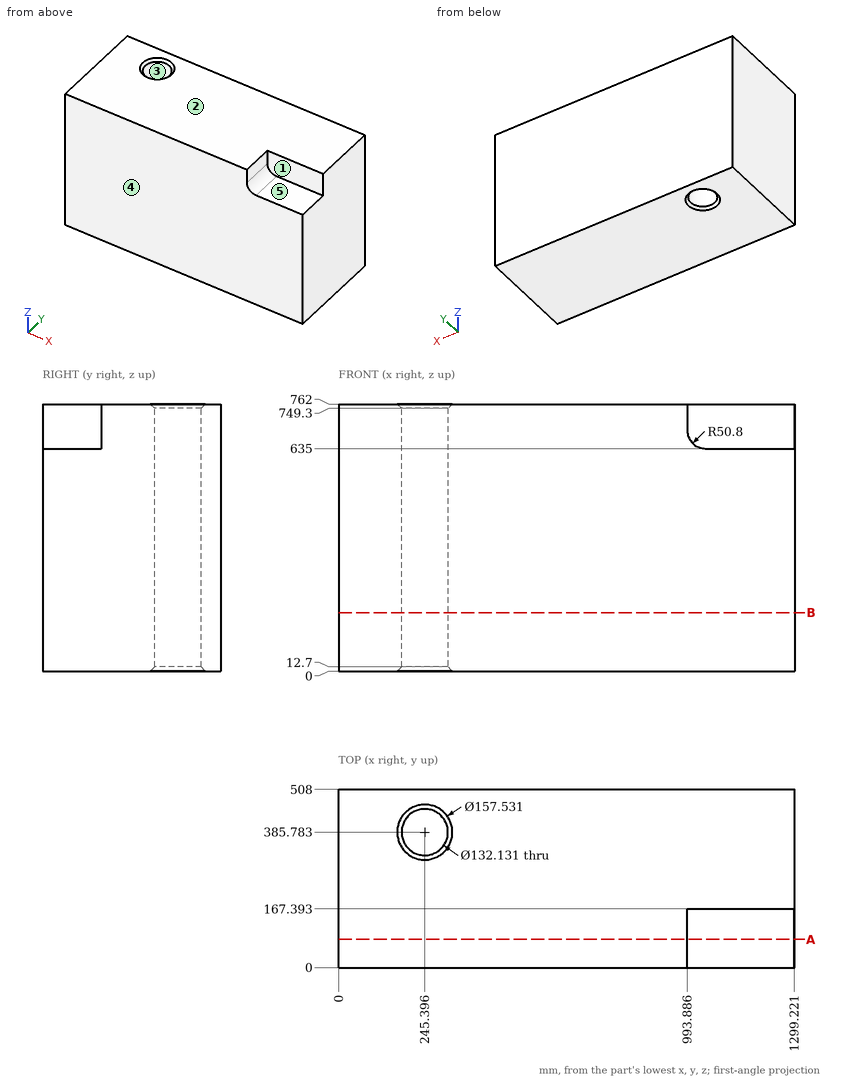
Design review of the part shown in the three views and the two pictorial views. Dimensions are in mm from the part's minimum x, y and z. A direction names the side the tool comes from. Coordinates: 2 decimals unless noted, no trailing zeros. Write each loop counter-clockwise with the first axis right and the second up, starting at its lowest first coordinate (ties: lowest second). Pieces come first, ordered by that corner, then holes.
(1) The part is to be moulded in two halves that separate along Y. For the marked faces 3, 4 and 5, say which applies: +Y half, -Y half, draft (parallel to the pull), parting line (faces both ways), or undercut.
(2) Wall thickness on probe 1 along Z at (x, y) = (1150.5, 45); probe 2 along X at (y, z) = (400, 229); probe 3 along X at (y, z) = (42, 704): over which ranges is each line inside the solid? List them lowest first.
(3) For pin 1 Ø5 at (y, z) = (113, 684.5) entering from -X; pin 2 Ø23 at (y, z) = (56, 739.5) entering from +X, all flat-tipped, find the tip position at first contact; note any pin that passes through.
(4) Add section B-B on z = 167. Give the boundary of the cut face in (x, y) (1 decimal), then the cut area to 3 significant figures.
(5) Add section A-A on y = 80.5. Give the boundary of the cut face in (x, z), then the cut area to 3 significant figures.
(6) Tool access review of the marked faces 1 and 2: name each direction out of +Z, -Z, +X, -X, +Y, -Y from which nothing blocks a thin tool from reaching the whole face with its end or side.
Answer sheet:
1. face 3: undercut
1. face 4: -Y half
1. face 5: draft
2. probe 1: z = 0 to 635
2. probe 2: x = 0 to 180.88, 309.91 to 1299.22
2. probe 3: x = 0 to 993.89
3. pin 1: stops at x = 0
3. pin 2: stops at x = 993.89
4. outline: (0, 0) - (1299.2, 0) - (1299.2, 508) - (0, 508) - close; hole circle Ø132.1 at (245.4, 385.8)
4. area: 646,000 mm2
5. outline: (0, 0) - (1299.22, 0) - (1299.22, 635) - (1044.69, 635) arc R50.8 cw to (993.89, 685.8) - (993.89, 762) - (0, 762) - close
5. area: 952,000 mm2
6. face 1: +Z, +X, -Y
6. face 2: +Z, +X, -X, +Y, -Y
